from build123d import *

# Parameters (mm, degrees)
F0_W     = 58.42
F0_H     = 66.3448
F0_R     = 1.3335
F1_DEPTH = 2.54
F2_W     = 16.51
F2_H     = 3.81
F3_DEPTH = 25.4


with BuildPart() as f1:
    # F0 (on Top) → F1 (new body)
    with BuildSketch(Plane.XY):
        with Locations((29.21, -33.1724)):
            Rectangle(F0_W, F0_H)
        with Locations((17.1196, -64.4398)):
            Circle(F0_R, mode=Mode.SUBTRACT)
        with Locations((41.3004, -64.4398)):
            Circle(F0_R, mode=Mode.SUBTRACT)
        with Locations((17.1196, -2.2098)):
            Circle(F0_R, mode=Mode.SUBTRACT)
        with Locations((41.3004, -2.2098)):
            Circle(F0_R, mode=Mode.SUBTRACT)
    extrude(amount=F1_DEPTH)

    # F2 (on face) → F3 (join)
    with BuildSketch(Plane.XY.offset(2.54)):
        with Locations((29.21, -1.905)):
            Rectangle(F2_W, F2_H)
    extrude(amount=F3_DEPTH)


solid = f1.part
Build history of the part. All positions in model axes, mm. A direction names the side the tool comes from. Round coordinates to 2 decimals unless told otherwise and drop trailing zeros. Write each loop counter-clockwise with the first axis right and the second up, starting at its lowest first coordinate (ties: lowest second). Pieces come first, ordered by that corner, then holes. Notation, with made-up numbers: M -21,-33.5 L 36,-33.5 A25 ccw 36,-14.5 Z; hole C 82.25,49.5 d11. An arc over 180 degrees is marked long. Use CSV: the item, a comma, the result in double quotes.
1. Saw through at B-B (z = 24). Give the cut face in (x, y) (3 decimals).
Reply:
outline,"M 20.955,-3.81 L 37.465,-3.81 L 37.465,0 L 20.955,0 Z"
2. Two-plate mould, pull along X, no slides. Class faces 1 (the face through (29, -2, 27.94)), 2 (the face through (17.735, -65.623, 1.252)), 3 (the face through (20.955, -2, 15)): +X half, -X half, draft (parallel to the pull), parting line (faces both ways), or undercut.
Reply:
face 1,"draft"
face 2,"undercut"
face 3,"-X half"
3. Tool access for faces 4 (the face through (0, -34, 1)), 5 (the face through (29, -3.81, 15)), 6 (the face through (37.465, -2, 15)): list every direction of +Z, -Z, +X, -X, +Y, -Y with a clear straight run to the whole face (end or side of a thin tool).
Reply:
face 4,"+Z, -Z, -X, +Y, -Y"
face 5,"+Z, +X, -X, -Y"
face 6,"+Z, +X, +Y, -Y"
4. Wall check: probe 1 along Z at (x, y) = (30, -13.5); probe 2 along Y at (x, z) = (35.5, 24.25); probe 3 along X at (y, z) = (-2.5, 10.5) (3 decimals). Give the ranges that are in metal, low to high. Write a range as from..to.
Reply:
probe 1,"z = 0..2.54"
probe 2,"y = -3.81..0"
probe 3,"x = 20.955..37.465"
5. Saw through at C-C (y = -24.5). Give the cut face in (x, z), plus the area to 3 significant figures.
Reply:
outline,"M 0,0 L 58.42,0 L 58.42,2.54 L 0,2.54 Z"
area,"148 mm²"
6. Saw through at A-A (x = 23.5). Give the cut face in (y, z).
Reply:
outline,"M -66.34,0 L 0,0 L 0,27.94 L -3.81,27.94 L -3.81,2.54 L -66.34,2.54 Z"
7. Flat gauge pins, fed straight in: pin 1 (13 mm diameter, centred on x = 29.5, z = 16.5, fed in from -Y); pin 2 (5 mm diameter, centred on x = 37.5, y = -40, fed in from -Z); pin 3 (3 mm diameter, centred on y = -2.5, z = 13, fed in from +X) (3 decimals); pin 4 (1.1 mm diameter, centred on y = -2, z = 19, fed in from -X) (3 decimals). Where does each tip first touch, or does it go through?
Reply:
pin 1,"stops at y = -3.81"
pin 2,"stops at z = 0"
pin 3,"stops at x = 37.465"
pin 4,"stops at x = 20.955"
